Build history of the part. All positions in model axes, mm. Face numbers are marked on the shaded views. A direction names the side the tool comes from. Coordinates: 2 decimals unless noted, no trailing zeros. Write each loop counter-clockwise with the first axis right and the second up, starting at its lowest first coordinate (ties: lowest second). Pieces come first, ordered by that corner, then holes.
Autodesk Inventor part; units mm, degrees
ref_plane "YZ Plane" through (0, 0, 0) normal (1, 0, 0) x (0, 1, 0)
ref_plane "XZ Plane" through (0, 0, 0) normal (0, 1, 0) x (-1, 0, 0)
ref_plane "XY Plane" through (0, 0, 0) normal (0, 0, 1) x (1, 0, 0)
sketch "Sketch2" plane through (0, 0, 0) normal (0, 0, 1) x (1, 0, 0)
  line L0 (0, 0) -> (10, 0)
  line L1 (10, 0) -> (0, 20)
  line L2 (0, 20) -> (0, 0)
  line L3 (0, 20) -> (0, 22.2361)
  line L4 (0, 22.2361) -> (11.118, 0)
  line L5 (10, 0) -> (11.118, 0)
  dimension "d4" = 20
  dimension "d8" = 1
  dimension "d9" = 10
revolve "Revolution1" add sketch "Sketch2" angle 360 about axis through (0, 20, 0) along (0, -1, 0) contours L1 L3 L4 L5
sketch "Sketch5" plane through (0, 0, 0) normal (0, -1, 0) x (1, 0, 0)
  circle A0 centre (0, 0) radius 10
  circle A1 centre (0, 0) radius 11.118
  circle A2 centre (0, 0) radius 11.118
  dimension "d11" = 20
extrude "Extrusion2" add sketch "Sketch5" along normal blind 10
sketch "Sketch7" plane through (0, 0, 0) normal (0, 1, 0) x (-1, 0, 0)
  circle A0 centre (0, 0) radius 1
  dimension "d14" = 2
extrude "Extrusion3" cut sketch "Sketch7" along normal up to surface
sketch "Sketch8" plane through (0, 0, 0) normal (0, 0, 1) x (1, 0, 0)
  line L0 (-1, 20.2361) -> (1, 20.2361)
  line L1 (-1, 20.2361) -> (-1, 35.2361)
  line L2 (-1, 35.2361) -> (-3, 35.2361)
  line L3 (-3, 35.2361) -> (-3, 15.9471)
  line L4 (-3, 15.9471) -> (-1, 20.2361)
  line L5 (0, 20.2361) -> (0, 25.2361)
  point P0 (0, 0)
  dimension "d17" = 115
  dimension "d18" = 2
  dimension "d20" = 15
revolve "Revolution2" add sketch "Sketch8" angle 360 about axis through (0, 20.2361, 0) along (0, 1, 0)
sketch "Sketch9" plane through (0, 0, 0) normal (1, 0, 0) x (0, 1, 0)
  circle A0 centre (26.2361, 0) radius 3
  line L0 (16.2361, 3) -> (16.2361, -3)
  point P0 (0, 0)
  dimension "d22" = 6
  dimension "d23" = 10
extrude "Extrusion4" add sketch "Sketch9" along normal mid plane 30
sketch "Sketch10" plane through (-15, 26.2361, 0) normal (-1, 0, 0) x (0, 0, 1)
  circle A0 centre (0, 0) radius 1
  circle A1 centre (0, 0) radius 3
  point P0 (0, -26.2361)
  dimension "d26" = 2
extrude "Extrusion5" cut sketch "Sketch10" against normal up to surface (30 mm away) contours A0
thread "Thread1"
thread "Thread2"
thread "Thread3"
sketch "Sketch11" plane through (0, 35.2361, 0) normal (0, 1, 0) x (1, 0, 0)
  circle A0 centre (0, 0) radius 1
extrude "Extrusion6" cut sketch "Sketch11" against normal blind 20
properties part number "Chemmix"
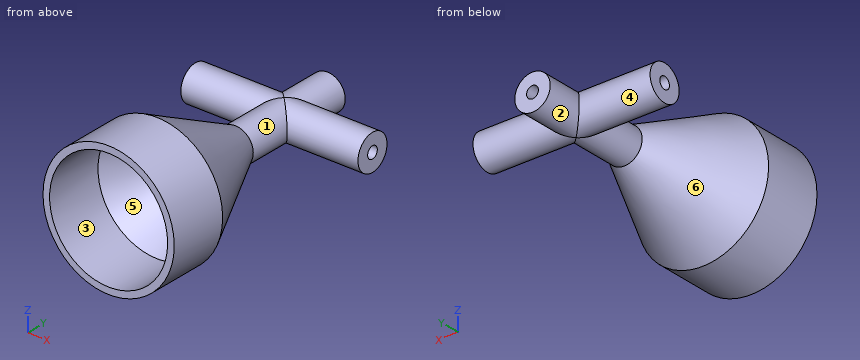
1. Mould opens along Z. For the marked faces 5 and 6 say: +Z half, -Z half, draft (parallel to the pull), parting line (faces both ways), or undercut.
Computed values:
face 5: undercut
face 6: parting line
2. Flat gauge pins, fed straight in: pin 1 (5 mm diameter, centred on y = 2, z = -9, fed in from -X); pin 2 (12 mm diameter, centred on x = 1.5, y = 18, fed in from +Z); pin 3 (4 mm diameter, centred on y = -3, z = -8.5, fed in from +X). Where does each tip first touch, or does it go through?
Computed values:
pin 1: stops at x = -8.31
pin 2: stops at z = 5.05
pin 3: stops at x = 9.02
3. Saw through at D-D on y = 6. List the corners of the cut face in (x, z).
Computed values:
outline: circle Ø16.24 at (0, 0); hole circle Ø14 at (0, 0)
4. Saw through at B-B on y = 21. List the corners of the cut face in (x, z), plus the area to 3 significant figures.
Computed values:
outline: circle Ø6 at (0, 0); hole circle Ø2 at (0, 0)
area: 25.1 mm2
5. Saw through at A-A on z = 0. State how many separate pieces and enclosed holes the cut face has, plus the area to 3 significant figures.
Computed values:
separate pieces: 4
enclosed holes: 0
area: 221 mm2
6. 3-axis set-ups, long thin cutter, end or side, ignore diameter. For the marked faces 1, 2, 3 and 4: which of +Z, -Z, +X, -X, +Y, -Y reach the whole face in a straight line?
Computed values:
face 1: none
face 2: +Y
face 3: -Y
face 4: -X
7. Probe line 1 along Y through (x, z) = (13, 0); line 2 along Y through (x, z) = (5, 0); line 3 along Y through (x, z) = (10.75, 0). List the from-to ranges inside material, lowest first.
Computed values:
line 1: y = 23.24 to 25.24, 27.24 to 29.24
line 2: y = 10 to 12.24, 23.24 to 25.24, 27.24 to 29.24
line 3: y = -10 to 0.74, 23.24 to 25.24, 27.24 to 29.24
